Check sheet for the modelled part. Datum: model origin and axes. Units: mm. A direction names the side the tool comes from. Give positions to 0.01 mm unless a question says otherwise; leave off trailing zeros. Order: outer loops, then holes, each group sorted by start corner. A loop starts at its lowest first (then second) coordinate and runs counter-clockwise, first axis right, second up.
from build123d import *

# Parameters (mm, degrees)
BOSS_EXTRUDE1_DEPTH = 100
SKETCH5_W           = 227.526539108
SKETCH5_H           = 7
BOSS_EXTRUDE4_DEPTH = 15
SKETCH6_W           = 7
SKETCH6_H           = 133
BOSS_EXTRUDE5_DEPTH = 15
FILLET2_R           = 60


with BuildPart() as part:
    # Sketch2 → Boss-Extrude1 (new body)
    with BuildSketch(Plane.XY):
        Polygon((-0.232315645, -1.10373444), (-50.232315645, -1.10373444), (-50.232315645, 148.89626556), (-48.232315645, 148.89626556), (-48.232315645, 0.89626556), (-3.293749688, 0.89626556), (-0.232315645, 0.89626556), (199.767684355, 0.89626556), (199.767684355, -1.10373444), align=None)
    extrude(amount=BOSS_EXTRUDE1_DEPTH)

    # Sketch5 → Boss-Extrude4 (add)
    with BuildSketch(Plane(origin=(0, 0.89626556, 0), x_dir=(1, 0, 0), z_dir=(0, 1, 0))):
        with Locations((65.530953909, -3.5)):
            Rectangle(SKETCH5_W, SKETCH5_H)
        with Locations((65.530953909, -96.5)):
            Rectangle(SKETCH5_W, SKETCH5_H)
    extrude(amount=BOSS_EXTRUDE4_DEPTH)

    # Sketch6 → Boss-Extrude5 (add)
    with BuildSketch(Plane(origin=(-48.232315645, 0, 0), x_dir=(0, 0, -1), z_dir=(1, 0, 0))):
        with Locations((-96.5, 82.39626556)):
            Rectangle(SKETCH6_W, SKETCH6_H)
        with Locations((-3.5, 82.39626556)):
            Rectangle(SKETCH6_W, SKETCH6_H)
    extrude(amount=BOSS_EXTRUDE5_DEPTH)

    # Fillet2
    fillet2_edges = [part.edges().sort_by_distance(p)[0] for p in [
        (-48.232315645, 0.89626556, 50),
        (-33.232315645, 15.89626556, 96.5),
        (-33.232315645, 15.89626556, 3.5),
    ]]
    fillet(fillet2_edges, radius=FILLET2_R)


solid = part.part
1) Section check A-A, the plane x = 40. Record the cut outline in (y, z).
Recorded:
outline: (-1.1, 0) - (15.9, 0) - (15.9, 7) - (0.9, 7) - (0.9, 93) - (15.9, 93) - (15.9, 100) - (-1.1, 100) - close
2) Depth check by flat-ended pin: pin 1 Ø5.5 at (x, z) = (103.5, 95) entering from +Y; pin 2 Ø3.5 at (y, z) = (6, 4.5) entering from +X; pin 3 Ø8 at (y, z) = (82.5, 30.5) entering from +X. Enter the tip coordinate at first touch or a pass-through.
Recorded:
pin 1: stops at y = 15.9
pin 2: stops at x = 179.29
pin 3: stops at x = -48.23
3) Set-up check for faces 1 (the face through (-50.232, 73, 49)), 2 (the face through (102, 15.896, 96)), 3 (the face through (-48.232, 106, 49)): record each of +Z, -Z, +X, -X, +Y, -Y from which the full face is reachable in a straight line by a thin tool's end or side.
Recorded:
face 1: +Z, -Z, -X, +Y, -Y
face 2: +Z, -Z, +X, +Y
face 3: +X, +Y
4) Material ranges on L1, parallel to Z at x = -30, y = 29; L2, parallel to Y at x = 187, z = 65; L3, parallel to X at y = 124, z = 95, recorded low to high.
Recorded:
L1: z = 0 to 7, 93 to 100
L2: y = -1.1 to 0.9
L3: x = -50.23 to -33.23
5) Section check B-B, the plane y = 136. Record the cut outline in (x, z), then the cut area to 3 significant figures.
Recorded:
outline: (-50.23, 0) - (-33.23, 0) - (-33.23, 7) - (-48.23, 7) - (-48.23, 93) - (-33.23, 93) - (-33.23, 100) - (-50.23, 100) - close
area: 410 mm2
6) Section check C-C, the plane z = 80. Record the cut outline in (x, y).
Recorded:
outline: (-50.23, -1.1) - (199.77, -1.1) - (199.77, 0.9) - (11.77, 0.9) arc R60 cw to (-48.23, 60.9) - (-48.23, 148.9) - (-50.23, 148.9) - close
